Input: part model. Units: mm. Frame: model coordinates. Give positions to 0.01 mm unless a question says otherwise; leave off trailing zeros. Write each loop counter-clockwise with the first axis right and the second up, starting at its lowest first coordinate (ties: lowest second). Pieces come first, ordered by that corner, then holes. Notation, with made-up numbers: (28, 58) - (53, 58) arc R17 cw to (53, 63) - close; hole circle Ø3 at (56, 65). An arc over 180 degrees is marked (long way). Answer as CSV lines item,"result". Start each with the question number.
from build123d import *

# Parameters (mm, degrees)
SKETCH2_R           = 2.54
SKETCH2_R_2         = 2.4892
BOSS_EXTRUDE4_DEPTH = 6.35


with BuildPart() as part:
    # Sketch2 → Boss-Extrude4 (new body)
    with BuildSketch(Plane.XY):
        with BuildLine():
            Line((16.553800999, 15.563538937), (-110.446199, 15.563538937))
            Line((-110.446199, 15.563538937), (-110.446199, 7.829313497))
            Line((-110.446199, 7.829313497), (8.327469614, 7.829313497))
            ThreePointArc((8.327469614, 7.829313497), (23.37971128, 6.58692566), (35.712064399, -2.132396173))
            ThreePointArc((35.712064399, -2.132396173), (58.549875935, -2.549801063), (55.400729061, 20.07369859))
            ThreePointArc((55.400729061, 20.07369859), (42.655168222, 22.428960004), (30.15762825, 18.992672461))
            ThreePointArc((30.15762825, 18.992672461), (23.568483326, 16.434024055), (16.553800999, 15.563538937))
        make_face()
        with Locations((52.410677776, 13.634120609)):
            Circle(SKETCH2_R, mode=Mode.SUBTRACT)
        with Locations((40, 2e-09)):
            Circle(SKETCH2_R_2, mode=Mode.SUBTRACT)
    extrude(amount=BOSS_EXTRUDE4_DEPTH)


solid = part.part
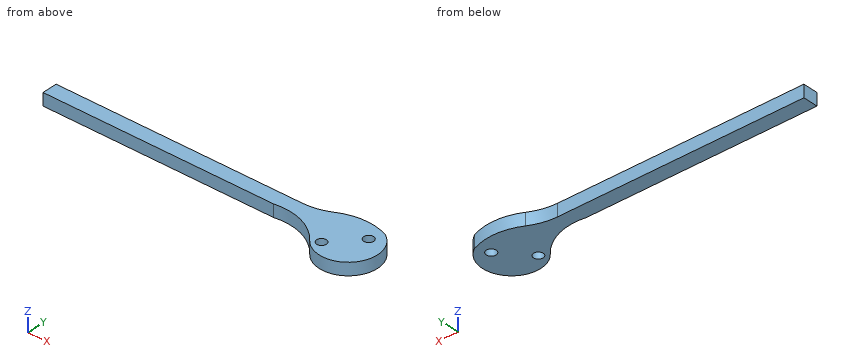
1) Cut plane A-A on x = 40. Output: boundary loops of the cut face in (y, z).
2) Cut plane B-B on z = 2.5. Output: boundary loops of the cut face in (x, y), and give its area (3 significant figures).
3) Contact query for flat-ended pins moving along their axis: P1, Ø8, axis at x = 7, y = 19.5, coming from the -Z side; P2, Ø4, axis at x = 52.41, y = 13.63, coming from the -Z side; P3, Ø1.9, axis at x = -42, z = 3.5, coming from the -Y side; P4, Ø1.5, axis at x = -7, z = 1.5, coming from the +Y side. Output: stop coordinate, or through.
4) Material intervals for line 1 (Y direction, x = -1, z = 5.25); line 2 (Y direction, x = 40, z = 1.5); line 3 (X direction, y = 15, z = 3.25), sorted ascending. Write a range as from..to.
5) Cut plane C-C on y = 0. Output: boundary loops of the cut face in (x, z), and give its area (3 significant figures).
6) Cut plane D-D on x = -7.5. Output: boundary loops of the cut face in (y, z).
Numbers:
1,outline,"(-5.71, 0) - (-2.49, 0) - (-2.49, 6.35) - (-5.71, 6.35) - close; (2.49, 0) - (22.19, 0) - (22.19, 6.35) - (2.49, 6.35) - close"
2,outline,"(-110.45, 7.83) - (8.33, 7.83) arc R28.67 cw to (35.71, -2.13) arc R15.02 ccw (long way) to (55.4, 20.07) arc R28.98 ccw to (30.16, 18.99) arc R28.7 cw to (16.55, 15.56) - (-110.45, 15.56) - close; hole circle Ø4.98 at (40, 0); hole circle Ø5.08 at (52.41, 13.63)"
2,area,"1,870 mm²"
3,P1,"stops at z = 0"
3,P2,"passes through"
3,P3,"stops at y = 7.83"
3,P4,"stops at y = 15.56"
4,line 1,"y = 7.83..15.56"
4,line 2,"y = -5.71..-2.49, 2.49..22.19"
4,line 3,"x = -110.45..50.27, 54.55..60.28"
5,outline,"(33.77, 0) - (37.51, 0) - (37.51, 6.35) - (33.77, 6.35) - close; (42.49, 0) - (60.37, 0) - (60.37, 6.35) - (42.49, 6.35) - close"
5,area,"137 mm²"
6,outline,"(7.83, 0) - (15.56, 0) - (15.56, 6.35) - (7.83, 6.35) - close"
